Geometry check sheet. Reference: drawing and pictorial views, mm from the part's lowest x, y, z. Give positions to 0.01 mm unless a question says otherwise; leave off trailing zeros. Order: outer loops, then holes, each group sorted by start corner. A loop starts at its lowest first (then second) coordinate and runs counter-clockwise, first axis right, second up. Notation, with made-up numbers: (31.25, -22.5) -> (76.25, -22.5) arc R19 cw to (76.25, -9.5) -> close; hole circle Ø3 at (-6.75, 85). An arc over 180 degrees is marked (long way). Write each question's results on one line, items separated by ' | '. Start each with the question number.
1. Depth check by flat-ended pin: pin 1 Ø2.5 at (x, y) = (25, 24.5) entering from -Z; pin 2 Ø6 at (x, y) = (19, 6.5) entering from -Z; pin 3 Ø10 at (y, z) = (16, 20.5) entering from -X; pin 4 Ø6 at (x, z) = (93, 22.5) entering from +Y. Enter the tip coordinate at first touch or a pass-through.
2. Cross-section at D-D, the plane z = 76.5. Enter the section's corners in (x, y).
3. Cross-section at B-B, the plane x = 96. Enter the section's corners in (y, z).
4. Cross-section at A-A, the plane y = 23.25. Enter the section's corners in (x, z).
5. Cross-section at C-C, the plane z = 104.5. Enter the section's corners in (x, y).
6. Material ranges on L1, parallel to Z at x = 96, y = 1.7; L2, parallel to X at y = 1.7, z = 24.5; L3, parallel to X at y = 4, z = 74.5, recorded low to high. Write a range as from..to.
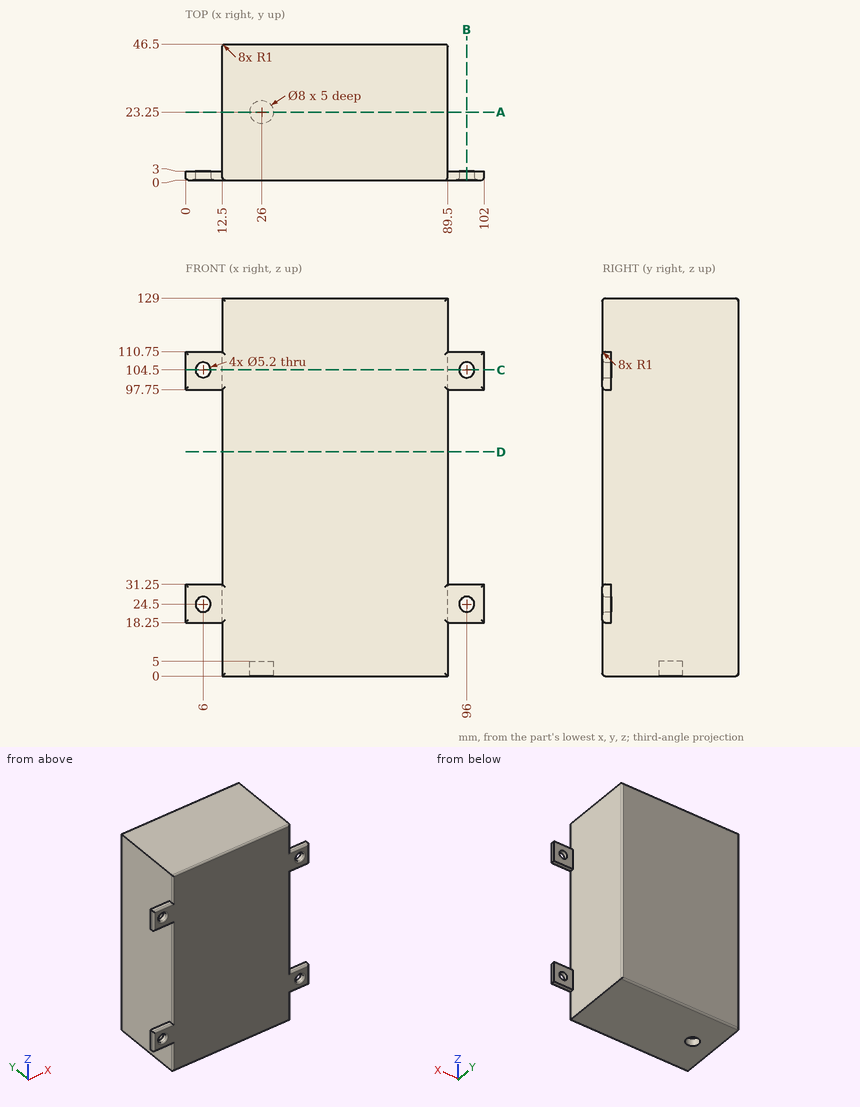
Results below:
1) pin 1: stops at z = 5 | pin 2: stops at z = 0 | pin 3: stops at x = 12.5 | pin 4: stops at y = 3
2) outline: (12.5, 1) arc R1 ccw to (13.5, 0) -> (88.5, 0) arc R1 ccw to (89.5, 1) -> (89.5, 45.5) arc R1 ccw to (88.5, 46.5) -> (13.5, 46.5) arc R1 ccw to (12.5, 45.5) -> close
3) outline: (0, 19.25) arc R1 ccw to (1, 18.25) -> (3, 18.25) -> (3, 21.9) -> (1, 21.9) arc R1 ccw to (0, 20.9) -> close; (0, 28.1) arc R1 ccw to (1, 27.1) -> (3, 27.1) -> (3, 31.25) -> (1, 31.25) arc R1 ccw to (0, 30.25) -> close; (0, 98.75) arc R1 ccw to (1, 97.75) -> (3, 97.75) -> (3, 101.9) -> (1, 101.9) arc R1 ccw to (0, 100.9) -> close; (0, 108.1) arc R1 ccw to (1, 107.1) -> (3, 107.1) -> (3, 110.75) -> (1, 110.75) arc R1 ccw to (0, 109.75) -> close
4) outline: (12.5, 0) -> (22, 0) -> (22, 5) -> (30, 5) -> (30, 0) -> (89.5, 0) -> (89.5, 129) -> (12.5, 129) -> close
5) outline: (0, 1) arc R1 ccw to (1, 0) -> (2.4, 0) arc R1 ccw to (3.4, 1) -> (3.4, 3) -> (0, 3) -> close; (8.6, 1) arc R1 ccw to (9.6, 0) -> (92.4, 0) arc R1 ccw to (93.4, 1) -> (93.4, 3) -> (89.5, 3) -> (89.5, 45.5) arc R1 ccw to (88.5, 46.5) -> (13.5, 46.5) arc R1 ccw to (12.5, 45.5) -> (12.5, 3) -> (8.6, 3) -> close; (98.6, 1) arc R1 ccw to (99.6, 0) -> (101, 0) arc R1 ccw to (102, 1) -> (102, 3) -> (98.6, 3) -> close
6) L1: z = 18.25..21.9, 27.1..31.25, 97.75..101.9, 107.1..110.75 | L2: x = 0..3.4, 8.6..93.4, 98.6..102 | L3: x = 12.5..89.5
